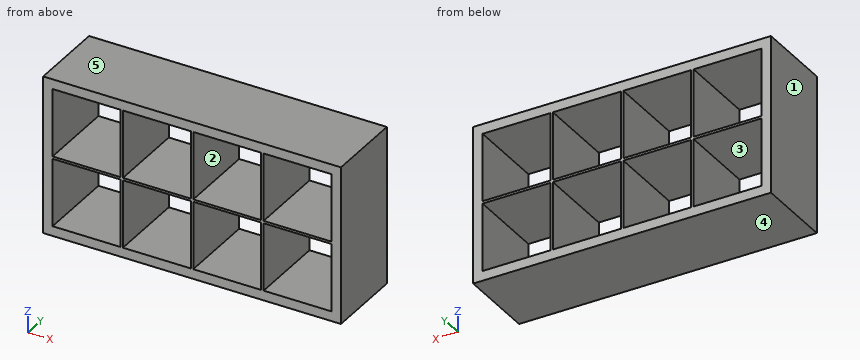
from build123d import *

# Parameters (mm, degrees)
F0_W     = 1490
F0_H     = 390
F1_DEPTH = 49
F2_W     = 47
F2_H     = 390
F2_W_2   = 12
F3_DEPTH = 692
F4_W     = 1490
F4_H     = 390
F5_DEPTH = 49
F6_W     = 390
F6_H     = 12
F7_DEPTH = 1410


with BuildPart() as f1:
    # F0 (on Top) → F1 (new body)
    with BuildSketch(Plane.XY):
        Rectangle(F0_W, F0_H)
    extrude(amount=F1_DEPTH)

    # F2 (on face) → F3 (join)
    with BuildSketch(Plane.XY.offset(49)):
        with Locations((-721.5, 0)):
            Rectangle(F2_W, F2_H)
        with Locations((721.5, 0)):
            Rectangle(F2_W, F2_H)
        with Locations((352, 0)):
            Rectangle(F2_W_2, F2_H)
        Rectangle(F2_W_2, F2_H)
        with Locations((-352, 0)):
            Rectangle(F2_W_2, F2_H)
    extrude(amount=F3_DEPTH)

    # F4 (on face) → F5 (join)
    with BuildSketch(Plane.XY.offset(741)):
        Rectangle(F4_W, F4_H)
    extrude(amount=F5_DEPTH)

    # F6 (on face) → F7 (join)
    with BuildSketch(Plane(origin=(698, 0, 0), x_dir=(0, -1, 0), z_dir=(-1, 0, 0))):
        with Locations((0, 395)):
            Rectangle(F6_W, F6_H)
    extrude(amount=F7_DEPTH)


solid = f1.part
Can you work these out from the model? Positions are in its coordinate system, mm. Face numbers are marked on the shaded views. A direction names the side the tool comes from. Give positions to 0.01 mm unless a question says otherwise; leave off trailing zeros. Order: outer loops, then holes, each group sorted by start corner. A loop starts at its lowest first (then second) coordinate and runs counter-clockwise, first axis right, second up. Notation, with made-up numbers: M 83,73 L 88,73 A19 cw 88,102 Z; hole C 86.5,17 d11. An arc over 180 degrees is marked long. Use one line per item in the form item = value. Start each with the question number.
Item 1: If we section it at A-A (x = 309.5): Write out the boundary of the cut face in (y, z).
Item 2: If we section it at C-C (y = 141.5): State how many separate pieces and enclosed holes the cut face has, then the cut area to 3 significant figures.
Item 3: For the marked faces 1 and 2, which set-ups out of +Z, -Z, +X, -X, +Y, -Y let a thin tool reach every point of the face, with its end or its side?
Item 4: If we section it at B-B (z = 416): Write out the boundary of the cut face in (x, y).
Item 5: If I drill on line 1 along Z through (x, y) = (629, -170.5); line 2 along X through (y, z) = (116.5, 74.5), over which ranges is the centre line in solid material (lowest first)?
Item 6: We'd pull the mould along Z, two halves only. Please class the marked faces 3, 4 and 5: +Z half, -Z half, draft (parallel to the pull), parting line (faces both ways), or undercut.
Outcome:
q1.outline = M -195,0 L 195,0 L 195,49 L -195,49 Z; M -195,389 L 195,389 L 195,401 L -195,401 Z; M -195,741 L 195,741 L 195,790 L -195,790 Z
q2.separate_pieces = 1
q2.enclosed_holes = 8
q2.area = 252,000 mm2
q3.face_1 = +Z, -Z, -X, +Y, -Y
q3.face_2 = +Y, -Y
q4.outline = M -745,-195 L -698,-195 L -698,195 L -745,195 Z; M -358,-195 L -346,-195 L -346,195 L -358,195 Z; M -6,-195 L 6,-195 L 6,195 L -6,195 Z; M 346,-195 L 358,-195 L 358,195 L 346,195 Z; M 698,-195 L 745,-195 L 745,195 L 698,195 Z
q5.line_1 = 0 to 49, 389 to 401, 741 to 790
q5.line_2 = -745 to -698, -358 to -346, -6 to 6, 346 to 358, 698 to 745
q6.face_3 = undercut
q6.face_4 = -Z half
q6.face_5 = +Z half
